Can you work these out from the model? Positions are in its coordinate system, mm. A direction names the side the tool comes from. Round coordinates to 2 decimals unless told otherwise and drop trailing zeros.
Autodesk Fusion 360 part; units mm, degrees
sketch "Sketch1" plane through (0, 0, 0) normal (0, 1, 0) x (1, 0, 0)
  line L0 (0, 0) -> (-35, 0)
  line L1 (0, 0) -> (0, -20)
  line L2 (0, -20) -> (-42, -20)
  arc A0 (-35, 0) -> (-42, -20) centre (-17.1273, -17.4804) ccw
  dimension "d1" = 35
  dimension "d2" = 20
  dimension "d3" = 42
  dimension "d4" = 25
revolve "Revolve1" add sketch "Sketch1" angle 360 about axis through (0, 0, 0) along (0, 0, 1)
sketch "Sketch2" plane through (0, 0, 20) normal (0, 0, 1) x (1, 0, 0)
  circle A0 centre (0, 0) radius 42
  circle A1 centre (0, 0) radius 39.5
  dimension "d6" = 79
extrude "Extrude1" add sketch "Sketch2" along normal blind 1 contours A1
sketch "Sketch4" plane through (0, 0, 21) normal (0, 0, 1) x (1, 0, 0)
  circle A0 centre (0, 0) radius 39.5
sketch "Sketch5" plane through (0, 0, 0) normal (0, 1, 0) x (1, 0, 0)
  line L0 (0, -21) -> (0, -41)
  line L1 (0, -41) -> (-42, -41)
  line L2 (0, -21) -> (-40, -21)
  arc A0 (-40, -21) -> (-42, -41) centre (-5.5677, -34.5432) ccw
  point P0 (0, -21)
  dimension "d9" = 20
  dimension "d10" = 42
  dimension "d11" = 40
  dimension "d12" = 37
revolve "Revolve2" add sketch "Sketch5" angle 360 about axis through (0, 0, 1.75) along (0, 0, 1)
sketch "Sketch6" plane through (0, 0, 41) normal (0, 0, 1) x (1, 0, 0)
  circle A0 centre (0, 0) radius 42
  circle A1 centre (0, 0) radius 41.25
  dimension "d14" = 82.5
extrude "Extrude2" add sketch "Sketch6" along normal blind 1 contours A1
(1) For faces 5 (the flat face through (-1, 1, 42)), 6 (the cylindrical face through (-29.11, -26.7, 20.49)), which set-ups out of +Z, -Z, +X, -X, +Y, -Y let a thin tool reach every point of the face, with its end or its side?
Worked answers:
face 5: +Z, +X, -X, +Y, -Y
face 6: none
(2) If we mould it in two halves opening along Z, with no side actions, what happens to faces 1 (the flat face through (-28, 31, 41)), 2 (the flat face through (0, 0, 0)), 3 (the flat face through (-25, 31, 20)), 4 (the cylindrical face through (-8.94, 40.27, 41.49))? For each: released by +Z, released by -Z, zero draft, split by the parting line, or undercut.
Worked answers:
face 1: released by +Z
face 2: released by -Z
face 3: undercut
face 4: zero draft
(3) Will these pins go through, and if not, where does the flat tip stop? P1, Ø1.5, axis at x = 23, z = 30.5, coming from the -Y side; P2, Ø12, axis at x = 24.5, z = 18, coming from the -Y side; P3, Ø10, axis at y = -2, z = 10, coming from the +X side.
Worked answers:
P1: stops at y = -36.04
P2: stops at y = -37.84
P3: stops at x = 41.98
(4) If I drill on line 1 (X direction, y = -24, z = 4); line 2 (Y direction, x = -35, z = 40.5); line 3 (Y direction, x = 4, z = 28), over which ranges is the centre line in solid material (lowest first)?
Worked answers:
line 1: x = -29.7 to 29.7
line 2: y = -23.37 to 23.37
line 3: y = -41.79 to 41.79
